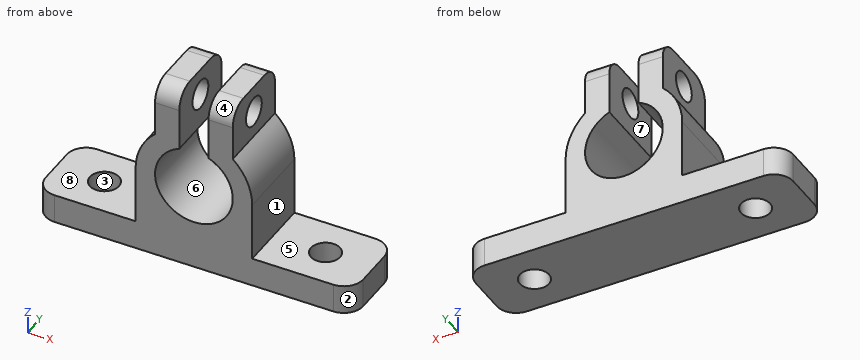
```python
from build123d import *

# Parameters (mm, degrees)
SKETCH_1_W          = 32.677388302
SKETCH_1_H          = 8
EXTRUDE_1_DEPTH     = 3
SKETCH_2_R          = 1.5
CUT_EXTRUDE_1_DEPTH = 4
SKETCH_3_R          = 6
EXTRUDE_2_DEPTH     = 8
SKETCH_4_R          = 4
CUT_EXTRUDE_2_DEPTH = 9
EXTRUDE_3_DEPTH     = 8
SKETCH_6_W          = 8
SKETCH_6_H          = 6
EXTRUDE_4_DEPTH     = 8
SKETCH_8_W          = 3
SKETCH_8_H          = 10.466633743
CUT_EXTRUDE_5_DEPTH = 9
SKETCH_9_R          = 1.5
CUT_EXTRUDE_6_DEPTH = 21.338694151
FILLET_1_R          = 2
FILLET_2_R          = 2


with BuildPart() as part:
    # Sketch 1 → Extrude 1 (new body)
    with BuildSketch(Plane.XY):
        with Locations((-3.726697353, 26.358574689)):
            Rectangle(SKETCH_1_W, SKETCH_1_H)
    extrude(amount=-EXTRUDE_1_DEPTH)

    # Sketch 2 → Cut-Extrude 1 (cut, through all)
    with BuildSketch(Plane.XY):
        with Locations((-15.101697353, 26.358574689)):
            Circle(SKETCH_2_R)
        with Locations((7.648302647, 26.358574689)):
            Circle(SKETCH_2_R)
    extrude(amount=-CUT_EXTRUDE_1_DEPTH, mode=Mode.SUBTRACT)



with BuildPart() as body_2:
    # Sketch 3 → Extrude 2 (new body)
    with BuildSketch(Plane.XZ.offset(-22.358574689)):
        with Locations((-3.726697353, 6)):
            Circle(SKETCH_3_R)
    extrude(amount=-EXTRUDE_2_DEPTH)

    # Sketch 4 → Cut-Extrude 2 (cut, through all)
    with BuildSketch(Plane.XZ.offset(-22.358574689)):
        with Locations((-3.726697353, 6)):
            Circle(SKETCH_4_R)
    extrude(amount=-CUT_EXTRUDE_2_DEPTH, mode=Mode.SUBTRACT)


with BuildPart() as part_1:
    add(part.part)

    add(body_2.part)  # Extrude 3 merges body 2
    # Sketch 5 → Extrude 3 (add)
    with BuildSketch(Plane.XZ.offset(-22.358574689)):
        Polygon((-3.726697353, 0), (-9.726697353, 6), (-9.726697353, 0), align=None)
        Polygon((2.273302647, 6), (-3.726697353, 0), (2.273302647, 0), align=None)
    extrude(amount=-EXTRUDE_3_DEPTH)

    # Sketch 6 → Extrude 4 (add)
    with BuildSketch(Plane.XZ.offset(-22.358574689)):
        with Locations((-3.726697353, 13)):
            Rectangle(SKETCH_6_W, SKETCH_6_H)
    extrude(amount=-EXTRUDE_4_DEPTH)

    # Sketch 8 → Cut-Extrude 5 (cut, through all)
    with BuildSketch(Plane.XZ.offset(-22.358574689)):
        with Locations((-3.726697353, 11.233316872)):
            Rectangle(SKETCH_8_W, SKETCH_8_H)
    extrude(amount=-CUT_EXTRUDE_5_DEPTH, mode=Mode.SUBTRACT)

    # Sketch 9 → Cut-Extrude 6 (cut, through all)
    with BuildSketch(Plane(origin=(0.273302647, 0, 0), x_dir=(0, 0, -1), z_dir=(1, 0, 0))):
        with Locations((-13.236067977, 26.358574689)):
            Circle(SKETCH_9_R)
    extrude(amount=-CUT_EXTRUDE_6_DEPTH, mode=Mode.SUBTRACT)

    # Fillet 1
    fillet_1_edges = [part_1.edges().sort_by_distance(p)[0] for p in [
        (12.611996798, 22.358574689, -1.5),
        (-20.065391504, 22.358574689, -1.5),
        (-20.065391504, 30.358574689, -1.5),
        (12.611996798, 30.358574689, -1.5),
    ]]
    fillet(fillet_1_edges, radius=FILLET_1_R)

    # Fillet 2
    fillet_2_edges = [part_1.edges().sort_by_distance(p)[0] for p in [
        (-0.976697353, 22.358574689, 16),
        (-0.976697353, 30.358574689, 16),
        (-6.476697353, 30.358574689, 16),
        (-6.476697353, 22.358574689, 16),
    ]]
    fillet(fillet_2_edges, radius=FILLET_2_R)


solid = part_1.part
```
Can you work these out from the model? Positions are in its coordinate system, mm. Face numbers are marked on the shaded views. A direction names the side the tool comes from. Round coordinates to 2 decimals unless told otherwise and drop trailing zeros. Loops run counter-clockwise (first coordinate to the right, second up) from the corner with the lowest first, then second, coordinate; pieces in that order, holes last. Notation, with made-up numbers: M 53,54 L 97,54 A4 ccw 97,60 Z; hole C -5.5,60.25 d5. An arc over 180 degrees is marked long. Answer as a JSON object with one key per item and string values. Group by question number.
Q1. Imagine slicing it at C-C, the plane y = 29.5. Please give me the cut outline in (x, z).
Q2. We'd pull the mould along Y, two halves only. Please class the marked faces 1, 2 and 3: +Y half, -Y half, draft (parallel to the pull), parting line (faces both ways), or undercut.
Q3. On a 3-axis mill with a long thin cutter (end or side, diameter ignored), from which of +Z, -Z, +X, -X, +Y, -Y can I reach the whole of each face in a straight line? I mean the marked faces 4, 5, 6, 7 and 8. Say none if no direction works.
Q4. Will these pins go through, and if not, where does the flat tip stop? pin 1 (3 mm diameter, centred on y = 26.5, z = 4, fed in from +X); pin 2 (2 mm diameter, centred on y = 28.5, z = 2, fed in from -X); pin 3 (6 mm diameter, centred on x = 3, z = 12, fed in from -Y); pin 4 (3 mm diameter, centred on y = 25, z = 13, fed in from +X).
Q5. Please list where these lines run through material, in increasing order: L1, parallel to X at y = 23.75, z = 14.75; L2, parallel to X at y = 28, z = 6; L3, parallel to Z at x = 10, y = 25.
Q6. Imagine slicing it at B-B, the plane z = 7.5. Please give me the cut outline in (x, y).
Q7. Imagine slicing it at D-D, the plane x = 3.5. Please give me the cut outline in (y, z).
Q8. Imagine slicing it at A-A, the plane x = -1. Please give me the cut outline in (y, z), then the cut area to 3 significant figures.
Findings:
{
 "1": {"outline": "M -19.71,-3 L 12.25,-3 L 12.25,0 L 2.27,0 L 2.27,6 A6 ccw 0.27,10.47 L 0.27,15.64 L -2.23,15.64 L -2.23,9.71 A4 cw long -5.23,9.71 L -5.23,15.64 L -7.73,15.64 L -7.73,10.47 A6 ccw -9.73,6 L -9.73,0 L -19.71,0 Z"},
 "2": {"face 1": "draft", "face 2": "-Y half", "face 3": "undercut"},
 "3": {"face 4": "+Z, +X, -X, -Y", "face 5": "+Z, +X, +Y, -Y", "face 6": "+Y, -Y", "face 7": "+Z, +Y, -Y", "face 8": "+Z, -X, +Y, -Y"},
 "4": {"pin 1": "stops at x = 2.27", "pin 2": "stops at x = -9.73", "pin 3": "stops at y = 22.36", "pin 4": "stops at x = 0.27"},
 "5": {"L1": "x = -7.73 to -5.23, -2.23 to 0.27", "L2": "x = -9.73 to -7.73, 0.27 to 2.27", "L3": "z = -3 to 0"},
 "6": {"outline": "M -9.54,22.36 L -7.43,22.36 L -7.43,30.36 L -9.54,30.36 Z; M -0.02,22.36 L 2.08,22.36 L 2.08,30.36 L -0.02,30.36 Z"},
 "7": {"outline": "M 22.36,-3 L 30.36,-3 L 30.36,0 L 22.36,0 Z"},
 "8": {"outline": "M 22.36,-3 L 30.36,-3 L 30.36,3.07 L 22.36,3.07 Z; M 22.36,8.93 L 30.36,8.93 L 30.36,14 A2 ccw 28.36,16 L 24.36,16 A2 ccw 22.36,14 Z; hole C 26.36,13.24 d3", "area": "96.4 mm2"}
}
